Can you work these out from the model? Positions are in its coordinate system, mm. Face numbers are marked on the shaded views. Round coordinates to 2 decimals unless told otherwise and drop trailing zeros. Order: outer loops, then holes, each group sorted by start corner. A loop starts at its lowest first (then second) coordinate and runs counter-clockwise, first axis right, second up.
Q1. If we section it at D-D (x = 2): Please give me the cut outline in (y, z).
Q2. Will these pins go through, and if not, where does the flat tip stop? P1, Ø5, axis at x = 10, y = 1, coming from the +Z side; P2, Ø8, axis at x = 12.5, z = 2.5, coming from the -Y side; P3, Ø4, axis at x = 6.5, y = -25.5, coming from the -Z side; P4, Ø5, axis at x = 12.5, z = 5.5, coming from the +Y side.
Q3. If we section it at C-C (x = 17.25): Please give me the cut outline in (y, z), plus the area to 3 significant figures.
Q4. If we section it at A-A (y = 0): Please give me the cut outline in (x, z) (3 decimals), plus the area to 3 significant figures.
Q5. If I drill on line 1 (Z direction, x = 7, y = 0); line 2 (Z direction, x = 21.75, y = 34.5); line 3 (Y direction, x = 16.5, z = -3), over which ranges is the centre line in solid material (lowest first)?
Q6. We'd pull the mould along Z, two halves only. Please class the marked faces 1, 2 and 3: pulls with the +Z half, pulls with the -Z half, needs draft (parallel to the pull), parting line crosses it, or undercut.
from build123d import *

# Parameters (mm, degrees)
F0_R     = 38.1
F0_R_2   = 6.35
F1_DEPTH = 25.908
F2_R     = 3.175
F3_SIZE  = 0.889


with BuildPart() as f1:
    # F0 (on Right) → F1 (new body)
    with BuildSketch(Plane.YZ):
        Circle(F0_R)
        Circle(F0_R_2, mode=Mode.SUBTRACT)
    extrude(amount=F1_DEPTH)

    # F2
    f2_edges = [f1.edges().sort_by_distance(p)[0] for p in [
        (12.954, 38.1, 0),
        (0, -38.1, 0),
        (25.908, -38.1, 0),
    ]]
    fillet(f2_edges, radius=F2_R)

    # F3
    f3_edges = [f1.edges().sort_by_distance(p)[0] for p in [
        (12.954, 6.35, 0),
        (0, -6.35, 0),
        (25.908, -6.35, 0),
    ]]
    chamfer(f3_edges, length=F3_SIZE)


solid = f1.part
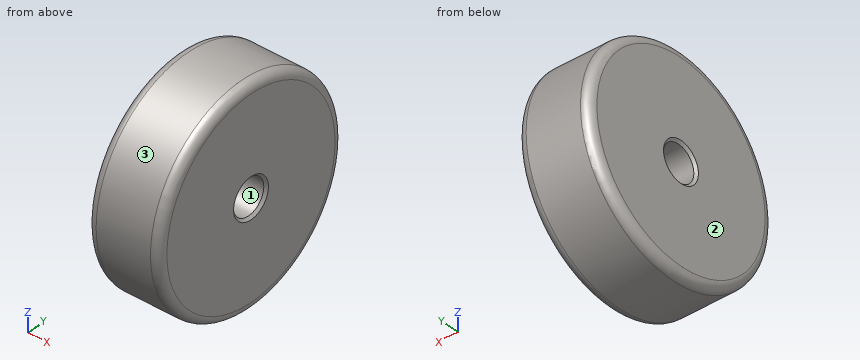
Solution:
1. outline: circle Ø75.75 at (0, 0); hole circle Ø12.7 at (0, 0)
2. P1: stops at z = 38.1
2. P2: stops at y = -38.1
2. P3: stops at z = -29.99
2. P4: stops at y = 37.98
3. outline: circle Ø76.2 at (0, 0); hole circle Ø12.7 at (0, 0)
3. area: 4,430 mm2
4. outline: (0, -34.925) arc R3.175 ccw to (3.175, -38.1) - (22.733, -38.1) arc R3.175 ccw to (25.908, -34.925) - (25.908, -7.239) - (25.019, -6.35) - (0.889, -6.35) - (0, -7.239) - close; (0, 7.239) - (0.889, 6.35) - (25.019, 6.35) - (25.908, 7.239) - (25.908, 34.925) arc R3.175 ccw to (22.733, 38.1) - (3.175, 38.1) arc R3.175 ccw to (0, 34.925) - close
4. area: 1,630 mm2
5. line 1: z = -38.1 to -6.35, 6.35 to 38.1
5. line 2: z = -16.17 to 16.17
5. line 3: y = -37.98 to -5.6, 5.6 to 37.98
6. face 1: undercut
6. face 2: needs draft
6. face 3: parting line crosses it
